from build123d import *
from build123d.topology import SkipClean

# Parameters (mm, degrees)
SKETCH1_R           = 60
SKETCH1_R_2         = 8
BOSS_EXTRUDE1_DEPTH = 4
BOSS_EXTRUDE2_DEPTH = 50
CUT_EXTRUDE1_DEPTH  = 47
SKETCH3_W           = 43.731073279
SKETCH3_H           = 43
CUT_EXTRUDE3_DEPTH  = 3


with BuildPart() as part:
    # Sketch1 → Boss-Extrude1 (new body)
    with BuildSketch(Plane.XY):
        Circle(SKETCH1_R)
        with BuildLine():
            Line((0.265819003, -56.90851166), (9.990859575, 0))
            Line((9.990859575, 0), (56.710923629, 0))
            ThreePointArc((56.710923629, 0), (40.206313594, -40.076778693), (0.265819003, -56.90851166))
        make_face(mode=Mode.SUBTRACT)
        Circle(SKETCH1_R_2, mode=Mode.SUBTRACT)
    extrude(amount=BOSS_EXTRUDE1_DEPTH)

    # Sketch1<3> → Boss-Extrude2 (add)
    with SkipClean():  # the faces are left unmerged after this step: merging them gives an invalid solid
        with BuildSketch(Plane.XY):
            with BuildLine():
                Line((60, 0), (9.990859575, 0))
                Line((9.990859575, 0), (-0.26238441, -59.999426284))
                ThreePointArc((-0.26238441, -59.999426284), (42.333538332, -42.519072571), (60, 0))
            make_face()
        extrude(amount=BOSS_EXTRUDE2_DEPTH)

    # Sketch1<6> → Cut-Extrude1 (cut)
    with SkipClean():  # the faces are left unmerged after this step: merging them gives an invalid solid
        with BuildSketch(Plane.XY):
            with BuildLine():
                ThreePointArc((3.3276834, -56.800985601), (41.2704357, -38.974638406), (56.710923629, 0))
                Line((56.710923629, 0), (13.034348947, 0))
                Line((13.034348947, 0), (12.521681846, -3))
                Line((12.521681846, -3), (3.3276834, -56.800985601))
            make_face()
        extrude(amount=CUT_EXTRUDE1_DEPTH, mode=Mode.SUBTRACT)

    # Sketch3 → Cut-Extrude3 (cut)
    with SkipClean():  # the faces are left unmerged after this step: merging them gives an invalid solid
        with BuildSketch(Plane(origin=(0, 0, 0), x_dir=(1, 0, 0), z_dir=(0, 1, 0))):
            with Locations((34.856396215, -25.5)):
                Rectangle(SKETCH3_W, SKETCH3_H)
        extrude(amount=-CUT_EXTRUDE3_DEPTH, mode=Mode.SUBTRACT)


solid = part.part
Source: CAD feature listing. Evaluate the final solid. Frame: model axes, mm. A direction names the side the tool comes from. Coordinates: 2 decimals unless noted, no trailing zeros. Loops run counter-clockwise (first coordinate to the right, second up) from the corner with the lowest first, then second, coordinate; pieces in that order, holes last. Notation, with made-up numbers: (-22, 66) -> (10, 66) arc R27 ccw to (10, 99) -> close; hole circle Ø7 at (-4.5, 71.25). An arc over 180 degrees is marked (long way). Answer in a Markdown table with one row per item. Add a question column.
Q1. Section B-B on x = 28.5. Return the cut outline in (y, z).
Q2. Section C-C on y = -45.5. Return the cut outline in (x, z).
Q3. Ray query, line 1 along Y through (x, z) = (0, 1.3); line 2 along Z through (x, y) = (-30, -18.5); line 3 along X through (y, z) = (-48, 36.5). Return the intervals inside material, ascending.
Q4. Contact query for flat-ended pins moving along their axis: pin 1 Ø3.5 at (y, z) = (-1.5, 30.5) entering from -X; pin 2 Ø6 at (y, z) = (-33.5, 12) entering from -X; pin 3 Ø2 at (x, z) = (44.5, 2.5) entering from -Y. Output: stop coordinate, or through.
Q5. Reachability of faces 1 (the face through (40.857, -39.41, 23.171)), 2 (the face through (35.1, 0, 47.3)) from +Z, -Z, +X, -X, +Y, -Y: full face, straight path, thin tool, end or side. Return the list, or none.
Q6. Section A-A on z = 27.5. Return the cut outline in (x, y), and give its area (3 significant figures).
Q7. Section D-D on x = 52.5. Return the cut outline in (y, z).
Q8. Pull-direction query (X, two-part tool) for faces 3 (the face through (-1, 14, 4)), 4 (the face through (35, 0, 2)), 5 (the face through (30, -22, 47)), 6 (the face through (4.936, -29.58, 26.678)); classes: pulls with the +X half, pulls with the -X half, needs draft (parallel to the pull), parting line crosses it, or undercut.
Computed values:
| question | item | result |
|---|---|---|
| 1 | outline | (-52.8, 0) -> (-49.14, 0) -> (-49.14, 47) -> (0, 47) -> (0, 50) -> (-52.8, 50) -> close; (0, 0) -> (52.8, 0) -> (52.8, 4) -> (0, 4) -> close |
| 2 | outline | (-39.11, 0) -> (5.26, 0) -> (5.26, 47) -> (33.98, 47) -> (33.98, 0) -> (39.11, 0) -> (39.11, 50) -> (2.22, 50) -> (2.22, 4) -> (-39.11, 4) -> close |
| 3 | line 1 | y = -60 to -8, 8 to 60 |
| 3 | line 2 | z = 0 to 4 |
| 3 | line 3 | x = 1.79 to 4.83, 30.37 to 36 |
| 4 | pin 1 | stops at x = 9.44 |
| 4 | pin 2 | stops at x = 3.75 |
| 4 | pin 3 | stops at y = -41.32 |
| 5 | face 1 | -Z |
| 5 | face 2 | +Z, +X, -X, +Y |
| 6 | outline | (-0.26, -60) arc R60 ccw to (60, 0) -> (56.72, 0) -> (56.72, -3) -> (56.63, -3) arc R56.91 cw to (3.33, -56.8) -> (12.99, -0.25) -> (12.99, 0) -> (9.99, 0) -> close |
| 6 | area | 468 mm^2 |
| 7 | outline | (-29.05, 0) -> (-21.48, 0) -> (-21.48, 47) -> (0, 47) -> (0, 50) -> (-29.05, 50) -> close; (0, 0) -> (29.05, 0) -> (29.05, 4) -> (0, 4) -> close |
| 8 | face 3 | needs draft |
| 8 | face 4 | undercut |
| 8 | face 5 | undercut |
| 8 | face 6 | pulls with the -X half |
